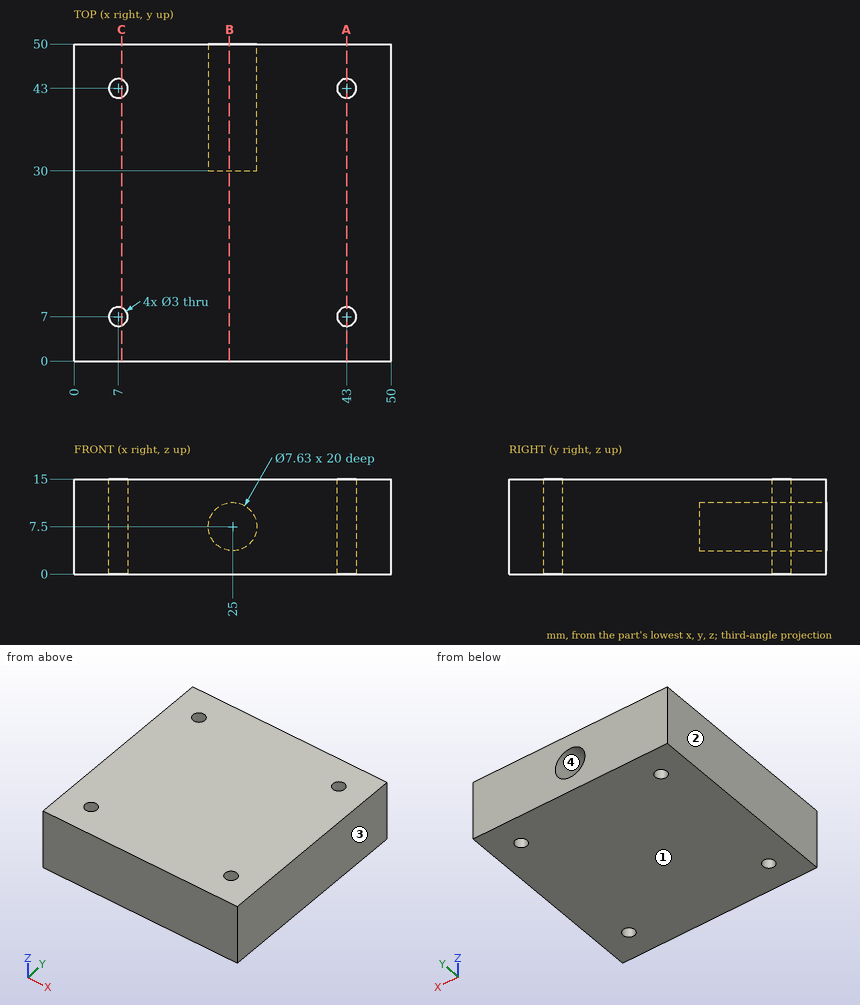
The figure shows three views and two pictorial views of one solid part (mm, origin at its lowest corner). Answer the questions. Round coordinates to 2 decimals unless told otherwise and drop trailing zeros. Loops run counter-clockwise (first coordinate to the right, second up) from the corner with the lowest first, then second, coordinate; pieces in that order, holes last. Notation, with made-up numbers: (-33, 53) -> (8, 53) arc R21 cw to (8, 63) -> close; hole circle Ø8 at (26.5, -37). An arc over 180 degrees is marked (long way). Use one line per item in the form item = value.
(1) Straight lines are drawn through the part: line 1 (Y direction, x = 7, z = 6); line 2 (X direction, y = 38, z = 5); line 3 (X direction, y = 35.5, z = 5.5). For each, find the intervals that lie inside material, in ascending order.
Answer list:
line_1 = 0 to 5.5, 8.5 to 41.5, 44.5 to 50
line_2 = 0 to 22.12, 27.88 to 50
line_3 = 0 to 21.75, 28.25 to 50
(2) Find section A-A on x = 43. Give the vertices of the cut face in (y, z).
Answer list:
outline = (0, 0) -> (5.5, 0) -> (5.5, 15) -> (0, 15) -> close; (8.5, 0) -> (41.5, 0) -> (41.5, 15) -> (8.5, 15) -> close; (44.5, 0) -> (50, 0) -> (50, 15) -> (44.5, 15) -> close
(3) Find section C-C on x = 7.5. Give the vertices of the cut face in (y, z).
Answer list:
outline = (0, 0) -> (5.59, 0) -> (5.59, 15) -> (0, 15) -> close; (8.41, 0) -> (41.59, 0) -> (41.59, 15) -> (8.41, 15) -> close; (44.41, 0) -> (50, 0) -> (50, 15) -> (44.41, 15) -> close
(4) For a pull along X with two mould halves and no side action, classify the marked faces 1, 2, 3 and 4 as released by +X, released by -X, zero draft, split by the parting line, or undercut.
Answer list:
face_1 = zero draft
face_2 = released by -X
face_3 = released by +X
face_4 = undercut
(5) Find section B-B on x = 24.5. Give the vertices of the cut face in (y, z), then the cut area to 3 significant figures.
Answer list:
outline = (0, 0) -> (50, 0) -> (50, 3.72) -> (30, 3.72) -> (30, 11.28) -> (50, 11.28) -> (50, 15) -> (0, 15) -> close
area = 599 mm2
